Geometry check sheet. Reference: the model listing, model coordinates, mm. Face numbers are marked on the shaded views. Coordinates: 2 decimals unless noted, no trailing zeros. Write each loop counter-clockwise with the first axis right and the second up, starting at its lowest first coordinate (ties: lowest second). Pieces come first, ordered by that corner, then holes.
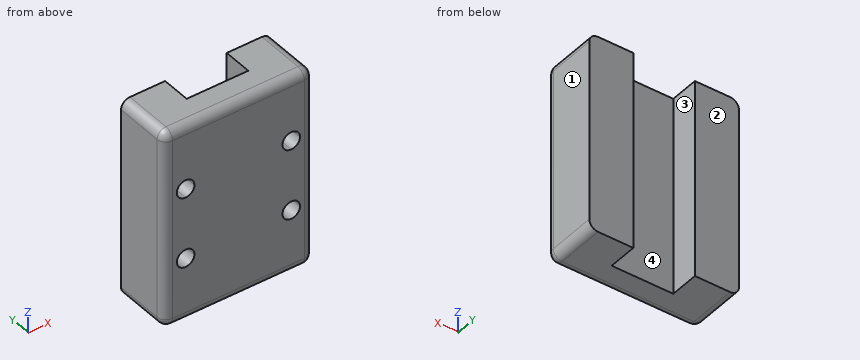
from build123d import *

# Parameters (mm, degrees)
EXTRUDE_1_DEPTH     = 22.5
CUT_EXTRUDE_1_DEPTH = 2.5
FILLET_1_R          = 1
FILLET_2_R          = 1


with BuildPart() as part:
    # 草图1 → 凸台-拉伸1 (new body)
    with BuildSketch(Plane.XY):
        Polygon((-8.5, 3.25), (-8.5, -3.25), (8.5, -3.25), (8.5, 3.25), (3.5, 3.25), (3.5, -0.05), (-3.5, -0.05), (-3.5, 3.25), align=None)
    extrude(amount=-EXTRUDE_1_DEPTH)

    # 草图2 → 切除-拉伸1 (cut)
    with BuildSketch(Plane.XZ.offset(3.25)):
        with BuildLine():
            Line((-6, -8.25), (-6, -7.25))
            Line((-6, -7.25), (-5, -7.25))
            ThreePointArc((-5, -7.25), (-6.707106781, -6.542893219), (-6, -8.25))
        make_face()
        with BuildLine():
            Line((-5, -7.25), (-6, -7.25))
            Line((-6, -7.25), (-6, -8.25))
            ThreePointArc((-6, -8.25), (-5.292893219, -7.957106781), (-5, -7.25))
        make_face()
        with BuildLine():
            ThreePointArc((7, -7.25), (6, -6.25), (5, -7.25))
            Line((5, -7.25), (6, -7.25))
            Line((6, -7.25), (6, -8.25))
            ThreePointArc((6, -8.25), (6.707106781, -7.957106781), (7, -7.25))
        make_face()
        with BuildLine():
            Line((6, -7.25), (5, -7.25))
            ThreePointArc((5, -7.25), (5.292893219, -7.957106781), (6, -8.25))
            Line((6, -8.25), (6, -7.25))
        make_face()
        with BuildLine():
            ThreePointArc((7, -15.25), (6.707106781, -14.542893219), (6, -14.25))
            Line((6, -14.25), (6, -15.25))
            Line((6, -15.25), (5, -15.25))
            ThreePointArc((5, -15.25), (6, -16.25), (7, -15.25))
        make_face()
        with BuildLine():
            Line((6, -15.25), (6, -14.25))
            ThreePointArc((6, -14.25), (5.292893219, -14.542893219), (5, -15.25))
            Line((5, -15.25), (6, -15.25))
        make_face()
        with BuildLine():
            ThreePointArc((-5, -15.25), (-5.292893219, -14.542893219), (-6, -14.25))
            Line((-6, -14.25), (-6, -15.25))
            Line((-6, -15.25), (-5, -15.25))
        make_face()
        with BuildLine():
            Line((-6, -15.25), (-6, -14.25))
            ThreePointArc((-6, -14.25), (-6.707106781, -15.957106781), (-5, -15.25))
            Line((-5, -15.25), (-6, -15.25))
        make_face()
    extrude(amount=-CUT_EXTRUDE_1_DEPTH, mode=Mode.SUBTRACT)

    # 圆角1
    fillet_1_edges = [part.edges().sort_by_distance(p)[0] for p in [
        (0, -3.25, 0),
        (8.5, -3.25, -11.25),
        (-8.5, -3.25, -11.25),
        (0, -3.25, -22.5),
    ]]
    fillet(fillet_1_edges, radius=FILLET_1_R)

    # 圆角2
    # the kernel refuses this fillet: 1 mm, written as the material it takes off along each edge
    with BuildSketch(Plane(origin=(-7.5, -2.25, -1), x_dir=(0, 0, 1), z_dir=(-1, 0, 0))) as fillet_2_piece_1_section:
        Polygon((0, 0), (FILLET_2_R, 0), (FILLET_2_R, -FILLET_2_R), (0, -FILLET_2_R), align=None)
    fillet_2_piece_1 = extrude(amount=FILLET_2_R, mode=Mode.PRIVATE)
    fillet_2_piece_1 = fillet_2_piece_1 - Plane(origin=(-7.5, -2.25, -1), x_dir=(0, 0.7071067811865475, -0.7071067811865475), z_dir=(-1, 0, 0)) * Sphere(FILLET_2_R, mode=Mode.PRIVATE)
    add(fillet_2_piece_1, mode=Mode.SUBTRACT)
    with BuildSketch(Plane(origin=(7.5, -2.25, -1), x_dir=(1, 0, 0), z_dir=(0, 0, 1))) as fillet_2_piece_2_section:
        Polygon((0, 0), (FILLET_2_R, 0), (FILLET_2_R, -FILLET_2_R), (0, -FILLET_2_R), align=None)
    fillet_2_piece_2 = extrude(amount=FILLET_2_R, mode=Mode.PRIVATE)
    fillet_2_piece_2 = fillet_2_piece_2 - Plane(origin=(7.5, -2.25, -1), x_dir=(-0.7071067811865475, 0.7071067811865475, 0), z_dir=(0, 0, 1)) * Sphere(FILLET_2_R, mode=Mode.PRIVATE)
    add(fillet_2_piece_2, mode=Mode.SUBTRACT)
    with BuildSketch(Plane(origin=(-7.5, -2.25, -21.5), x_dir=(0, 0, -1), z_dir=(-1, 0, 0))) as fillet_2_piece_3_section:
        Polygon((0, 0), (FILLET_2_R, 0), (FILLET_2_R, FILLET_2_R), (0, FILLET_2_R), align=None)
    fillet_2_piece_3 = extrude(amount=FILLET_2_R, mode=Mode.PRIVATE)
    fillet_2_piece_3 = fillet_2_piece_3 - Plane(origin=(-7.5, -2.25, -21.5), x_dir=(0, 0.7071067811865475, 0.7071067811865475), z_dir=(-1, 0, 0)) * Sphere(FILLET_2_R, mode=Mode.PRIVATE)
    add(fillet_2_piece_3, mode=Mode.SUBTRACT)
    with BuildSketch(Plane(origin=(7.5, -2.25, -21.5), x_dir=(1, 0, 0), z_dir=(0, 0, -1))) as fillet_2_piece_4_section:
        Polygon((0, 0), (FILLET_2_R, 0), (FILLET_2_R, FILLET_2_R), (0, FILLET_2_R), align=None)
    fillet_2_piece_4 = extrude(amount=FILLET_2_R, mode=Mode.PRIVATE)
    fillet_2_piece_4 = fillet_2_piece_4 - Plane(origin=(7.5, -2.25, -21.5), x_dir=(-0.7071067811865475, 0.7071067811865475, 0), z_dir=(0, 0, -1)) * Sphere(FILLET_2_R, mode=Mode.PRIVATE)
    add(fillet_2_piece_4, mode=Mode.SUBTRACT)
    with BuildSketch(Plane(origin=(8.5, -2.25, -22.5), x_dir=(-1, 0, 0), z_dir=(0, 1, 0)), Plane(origin=(-8.5, 5.75, 0), x_dir=(0, 0, -1), z_dir=(0, -1, 0))) as fillet_2_piece_5:
        with BuildLine():
            CenterArc((FILLET_2_R, FILLET_2_R), FILLET_2_R, 180, 90)
            Line((0, FILLET_2_R), (0, 0))
            Line((0, 0), (FILLET_2_R, 0))
        make_face()
    extrude(amount=8, mode=Mode.SUBTRACT)
    with BuildSketch(Plane(origin=(-8.5, 5.75, -22.5), x_dir=(0, 0, 1), z_dir=(0, -1, 0)), Plane(origin=(8.5, -2.25, 0), x_dir=(-1, 0, 0), z_dir=(0, 1, 0))) as fillet_2_piece_6:
        with BuildLine():
            CenterArc((FILLET_2_R, -FILLET_2_R), FILLET_2_R, 90, 90)
            Line((0, -FILLET_2_R), (0, 0))
            Line((0, 0), (FILLET_2_R, 0))
        make_face()
    extrude(amount=8, mode=Mode.SUBTRACT)


solid = part.part
1. Sectioned sample at B-B, the plane z = -2.75. Record the boundary of the cut face in (x, y).
Computed values:
outline: (-8.5, -2.25) arc R1 ccw to (-7.5, -3.25) - (7.5, -3.25) arc R1 ccw to (8.5, -2.25) - (8.5, 3.25) - (3.5, 3.25) - (3.5, -0.05) - (-3.5, -0.05) - (-3.5, 3.25) - (-8.5, 3.25) - close
2. Gauge pin test, flat ends, axial feed: pin 1 Ø5.5 at (x, z) = (0, -16.5) entering from +Y; pin 2 Ø1.8 at (x, z) = (-6, -7.25) entering from -Y. Record the tip position at first contact, or that the pin passes through.
Computed values:
pin 1: stops at y = -0.05
pin 2: stops at y = -0.75
3. Thickness scan on line 1 along X through (y, z) = (-1.9, -15.25); line 2 along Z through (x, y) = (-6, -2.2); line 3 along X through (y, z) = (0.5, -15.5). Record the ranges inside material, lowest first.
Computed values:
line 1: x = -8.5 to -7, -5 to 5, 7 to 8.5
line 2: z = -22.5 to -16.25, -14.25 to -8.25, -6.25 to 0
line 3: x = -8.5 to -3.5, 3.5 to 8.5
4. Sectioned sample at A-A, the plane y = 2.25. Record the boundary of the cut face in (x, z), and give its area (3 significant figures).
Computed values:
outline: (-8.5, -21.5) arc R1 ccw to (-7.5, -22.5) - (-3.5, -22.5) - (-3.5, 0) - (-7.5, 0) arc R1 ccw to (-8.5, -1) - close; (3.5, -22.5) - (7.5, -22.5) arc R1 ccw to (8.5, -21.5) - (8.5, -1) arc R1 ccw to (7.5, 0) - (3.5, 0) - close
area: 224 mm2
5. Sectioned sample at D-D, the plane x = 0.25. Record the boundary of the cut face in (y, z), and give its area (3 significant figures).
Computed values:
outline: (-3.25, -21.5) arc R1 ccw to (-2.25, -22.5) - (-0.05, -22.5) - (-0.05, 0) - (-2.25, 0) arc R1 ccw to (-3.25, -1) - close
area: 71.6 mm2
6. Sectioned sample at C-C, the plane y = -3. Record the boundary of the cut face in (x, z), and give its area (3 significant figures).
Computed values:
outline: (-8.16, -21.5) arc R0.66 ccw to (-7.5, -22.16) - (7.5, -22.16) arc R0.66 ccw to (8.16, -21.5) - (8.16, -1) arc R0.66 ccw to (7.5, -0.34) - (-7.5, -0.34) arc R0.66 ccw to (-8.16, -1) - close; hole circle Ø2 at (-6, -15.25); hole circle Ø2 at (-6, -7.25); hole circle Ø2 at (6, -15.25); hole circle Ø2 at (6, -7.25)
area: 343 mm2
7. Draft check along X on the marked faces 1, 2, 3 and 4. Enter one of: released by +X, released by -X, zero draft, split by the parting line, or undercut.
Computed values:
face 1: released by +X
face 2: zero draft
face 3: undercut
face 4: undercut
